The figure shows three views and two pictorial views of one solid part (mm, origin at its lowest corner). Answer the questions. A direction names the side the tool comes from. Coordinates: 2 decimals unless noted, no trailing zeros. Write each loop counter-clockwise with the first axis right and the second up, starting at its lowest first coordinate (ties: lowest second). Pieces come first, ordered by that corner, then holes.
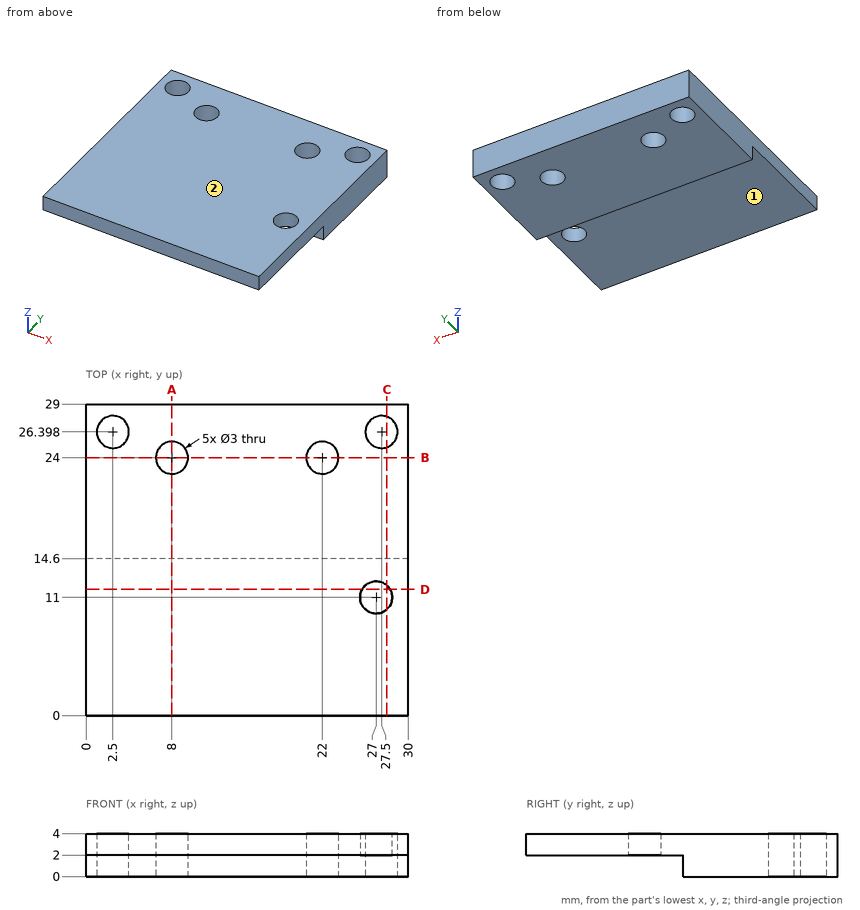
1. Section B-B on y = 24 is taken. Give the vertices of the cut face in (x, z).
Results found:
outline: (0, 0) - (6.5, 0) - (6.5, 4) - (0, 4) - close; (9.5, 0) - (20.5, 0) - (20.5, 4) - (9.5, 4) - close; (23.5, 0) - (30, 0) - (30, 4) - (23.5, 4) - close
2. Section D-D on y = 11.75 is taken. Give the vertices of the cut face in (x, z), then the cut area to 3 significant figures.
Results found:
outline: (0, 2) - (25.7, 2) - (25.7, 4) - (0, 4) - close; (28.3, 2) - (30, 2) - (30, 4) - (28.3, 4) - close
area: 54.8 mm2
3. Find the intervals of material crossed by L1, parallel to Y at x = 27.5, z = 1.3; L2, parallel to X at y = 11, z = 3.3; L3, parallel to Z at x = 18, y = 5.5, in increasing order.
Results found:
L1: y = 14.6 to 24.9, 27.9 to 29
L2: x = 0 to 25.5, 28.5 to 30
L3: z = 2 to 4
4. Section A-A on x = 8 is taken. Give the vertices of the cut face in (y, z), then the cut area to 3 significant figures.
Results found:
outline: (0, 2) - (14.6, 2) - (14.6, 0) - (22.5, 0) - (22.5, 4) - (0, 4) - close; (25.5, 0) - (29, 0) - (29, 4) - (25.5, 4) - close
area: 74.8 mm2
5. A tool of negligible diameter and unlimited length cuts with its end or side. For the marked faces 1 and 2, from which of +Z, -Z, +X, -X, +Y, -Y can it reach the whole face along a straight path? Write none if from no direction.
Results found:
face 1: -Z, +X, -X, -Y
face 2: +Z, +X, -X, +Y, -Y
6. Section C-C on x = 28 is taken. Give the vertices of the cut face in (y, z).
Results found:
outline: (0, 2) - (9.88, 2) - (9.88, 4) - (0, 4) - close; (12.12, 2) - (14.6, 2) - (14.6, 0) - (24.98, 0) - (24.98, 4) - (12.12, 4) - close; (27.81, 0) - (29, 0) - (29, 4) - (27.81, 4) - close
7. Flat-ended cylindrical pins translate along their axes: P1, Ø1, axis at x = 10.5, z = 1, coming from the -Y side; P2, Ø11.5, axis at x = 18, y = 4, coming from the -Z side. Find the tip coordinate at first contact, or state that the pin passes through.
Results found:
P1: stops at y = 14.6
P2: stops at z = 2
